Could you check a few things on this model? Use its own coordinates, in mm. A direction names the side the tool comes from. Round coordinates to 2 decimals unless told otherwise and drop trailing zeros. Order: outer loops, then holes, each group sorted by start corner. A loop starts at its lowest first (then second) coordinate and runs counter-clockwise, first axis right, second up. Notation, with made-up numbers: (35, 23.25) - (59, 23.25) arc R31 ccw to (59, 50.25) - close; hole circle Ø11 at (-26, 79). An arc over 180 degrees is marked (long way). Use one line per item in the form item = value.
from build123d import *

# Parameters (mm, degrees)
F1_DEPTH = 20
F2_R     = 10
F3_DEPTH = 20


with BuildPart() as f1:
    # F0 (on Front) → F1 (new body)
    with BuildSketch(Plane.XZ):
        with BuildLine():
            ThreePointArc((-9.682458, 62.5), (-1.260043, 50.079703), (10, 60))
            ThreePointArc((10, 60), (9.920297, 61.260043), (9.682458, 62.5))
            ThreePointArc((9.682458, 62.5), (0, 70), (-9.682458, 62.5))
        make_face()
        with BuildLine():
            ThreePointArc((9.682458, 62.5), (9.920297, 61.260043), (10, 60))
            ThreePointArc((10, 60), (-1.260043, 50.079703), (-9.682458, 62.5))
            Line((-9.682458, 62.5), (-24.206146, 6.25))
            ThreePointArc((-24.206146, 6.25), (0, 25), (24.206146, 6.25))
            Line((24.206146, 6.25), (9.682458, 62.5))
        make_face()
        with BuildLine():
            ThreePointArc((25, 0), (24.800742, 3.150107), (24.206146, 6.25))
            ThreePointArc((24.206146, 6.25), (0, 25), (-24.206146, 6.25))
            ThreePointArc((-24.206146, 6.25), (-3.150107, -24.800742), (25, 0))
        make_face()
    extrude(amount=F1_DEPTH)

    # F2 (on face) → F3 (join)
    with BuildSketch(Plane.XZ.offset(20)):
        Circle(F2_R)
    extrude(amount=F3_DEPTH)


solid = f1.part
Item 1: Imagine slicing it at A-A on x = 0. Please give me the cut outline in (y, z), plus the area to 3 significant figures.
Found:
outline = (-40, -10) - (-20, -10) - (-20, -25) - (0, -25) - (0, 70) - (-20, 70) - (-20, 10) - (-40, 10) - close
area = 2,300 mm2
Item 2: Imagine slicing it at D-D on y = -32.5. Please give me the cut outline in (x, z).
Found:
outline = circle Ø20 at (0, 0)
Item 3: Will these pins go through, and if not, where does the flat tip stop? P1, Ø8, axis at y = -7.5, z = 13.5, coming from the -X side; P2, Ø5, axis at x = -8.5, z = 51.5, coming from the -Y side; P3, Ø3, axis at y = -16, z = 16.5, coming from the -X side.
Found:
P1 = -23.37
P2 = -20
P3 = -21.95
Item 4: Imagine slicing it at B-B on y = -7.5. Please give me the cut outline in (x, z).
Found:
outline = (-24.21, 6.25) arc R25 ccw (long way) to (25, 0) arc R25 ccw to (24.21, 6.25) - (9.68, 62.5) arc R10 ccw to (-9.68, 62.5) - close
Item 5: For faces 1 (the face through (-2.17, -29.86, -9.76)), 2 (the face through (0, -10, 70)), which set-ups out of +Z, -Z, +X, -X, +Y, -Y let a thin tool reach every point of the face, with its end or its side?
Found:
face_1 = -Y
face_2 = +Z, +Y, -Y
Item 6: Imagine slicing it at C-C on x = -7. Please give me the cut outline in (y, z).
Found:
outline = (-40, -7.14) - (-20, -7.14) - (-20, -24) - (0, -24) - (0, 67.14) - (-20, 67.14) - (-20, 7.14) - (-40, 7.14) - close
Item 7: I need wall thicknesses on L1, parallel to Y at x = -20.5, z = -2; L2, parallel to Z at x = -2.5, y = -27; L3, parallel to Z at x = -0.5, y = -27. Which ranges of each line are inside material? Lowest first, please.
Found:
L1 = -20 to 0
L2 = -9.68 to 9.68
L3 = -9.99 to 9.99
